from build123d import *

# Parameters (mm, degrees)
EXTRUDE_1_DEPTH     = 1500
CUT_EXTRUDE_4_DEPTH = 1500
SHELL_3_T           = 10


with BuildPart() as part:
    # 草图2 → 凸台-拉伸1 (new body)
    with BuildSketch(Plane(origin=(0, 0, 0), x_dir=(1, 0, 0), z_dir=(0, 1, 0))):
        Polygon((345, 8.660254038), (180, 294.448637287), (165, 303.108891325), (-165, 303.108891325), (-180, 294.448637287), (-345, 8.660254038), (-345, -8.660254038), (-180, -294.448637287), (-165, -303.108891325), (165, -303.108891325), (180, -294.448637287), (345, -8.660254038), align=None)
    extrude(amount=EXTRUDE_1_DEPTH)

    # 草图5 → 切除-拉伸4 (cut)
    with BuildSketch(Plane(origin=(0, 0, 0), x_dir=(1, 0, 0), z_dir=(0, 1, 0))):
        with BuildLine():
            Line((165, 303.108891325), (16.245071573, 258.879313504))
            ThreePointArc((16.245071573, 258.879313504), (0, 256.515365505), (-16.245071573, 258.879313504))
            Line((-16.245071573, 258.879313504), (-165, 303.108891325))
            Line((-165, 303.108891325), (-165, 323.92213511))
            Line((-165, 323.92213511), (-16.245047342, 368.151648331))
            ThreePointArc((-16.245047342, 368.151648331), (0, 370.515589126), (16.245047342, 368.151648331))
            Line((16.245047342, 368.151648331), (165, 323.92213511))
            Line((165, 323.92213511), (165, 303.108891325))
        make_face()
        with BuildLine():
            Line((198.024797853, 304.855259179), (310.706156229, 198.14444785))
            ThreePointArc((310.706156229, 198.14444785), (320.875912682, 185.257794563), (326.951203571, 170.007200482))
            Line((326.951203571, 170.007200482), (363.024797853, 19.06687593))
            Line((363.024797853, 19.06687593), (345, 8.660254038))
            Line((345, 8.660254038), (232.318597795, 115.371012084))
            ThreePointArc((232.318597795, 115.371012084), (222.148822988, 128.257682752), (216.073526222, 143.50830142))
            Line((216.073526222, 143.50830142), (180, 294.448637287))
            Line((180, 294.448637287), (198.024797853, 304.855259179))
        make_face()
        with BuildLine():
            Line((363.024797853, -19.06687593), (326.951203571, -170.007200482))
            ThreePointArc((326.951203571, -170.007200482), (320.875912682, -185.257794563), (310.706156229, -198.14444785))
            Line((310.706156229, -198.14444785), (198.024797853, -304.855259179))
            Line((198.024797853, -304.855259179), (180, -294.448637287))
            Line((180, -294.448637287), (216.073526222, -143.50830142))
            ThreePointArc((216.073526222, -143.50830142), (222.148822988, -128.257682752), (232.318597795, -115.371012084))
            Line((232.318597795, -115.371012084), (345, -8.660254038))
            Line((345, -8.660254038), (363.024797853, -19.06687593))
        make_face()
        with BuildLine():
            Line((165, -323.92213511), (16.245047342, -368.151648331))
            ThreePointArc((16.245047342, -368.151648331), (0, -370.515589126), (-16.245047342, -368.151648331))
            Line((-16.245047342, -368.151648331), (-165, -323.92213511))
            Line((-165, -323.92213511), (-165, -303.108891325))
            Line((-165, -303.108891325), (-16.245071573, -258.879313504))
            ThreePointArc((-16.245071573, -258.879313504), (0, -256.515365505), (16.245071573, -258.879313504))
            Line((16.245071573, -258.879313504), (165, -303.108891325))
            Line((165, -303.108891325), (165, -323.92213511))
        make_face()
        with BuildLine():
            Line((-198.024797853, -304.855259179), (-310.706156229, -198.14444785))
            ThreePointArc((-310.706156229, -198.14444785), (-320.875912682, -185.257794563), (-326.951203571, -170.007200482))
            Line((-326.951203571, -170.007200482), (-363.024797853, -19.06687593))
            Line((-363.024797853, -19.06687593), (-345, -8.660254038))
            Line((-345, -8.660254038), (-232.318597795, -115.371012084))
            ThreePointArc((-232.318597795, -115.371012084), (-222.148822988, -128.257682752), (-216.073526222, -143.50830142))
            Line((-216.073526222, -143.50830142), (-180, -294.448637287))
            Line((-180, -294.448637287), (-198.024797853, -304.855259179))
        make_face()
        with BuildLine():
            Line((-363.024797853, 19.06687593), (-326.951203571, 170.007200482))
            ThreePointArc((-326.951203571, 170.007200482), (-320.875912682, 185.257794563), (-310.706156229, 198.14444785))
            Line((-310.706156229, 198.14444785), (-198.024797853, 304.855259179))
            Line((-198.024797853, 304.855259179), (-180, 294.448637287))
            Line((-180, 294.448637287), (-216.073526222, 143.50830142))
            ThreePointArc((-216.073526222, 143.50830142), (-222.148822988, 128.257682752), (-232.318597795, 115.371012084))
            Line((-232.318597795, 115.371012084), (-345, 8.660254038))
            Line((-345, 8.660254038), (-363.024797853, 19.06687593))
        make_face()
    extrude(amount=CUT_EXTRUDE_4_DEPTH, mode=Mode.SUBTRACT)

    # 抽壳3 (no face opened: a closed hollow body)
    add(offset(amount=-SHELL_3_T, mode=Mode.PRIVATE), mode=Mode.SUBTRACT)


solid = part.part
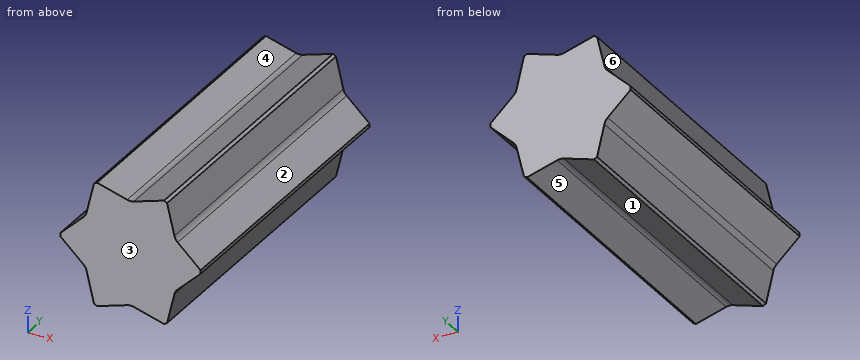
Geometry check sheet. Reference: the model listing, model coordinates, mm. Face numbers are marked on the shaded views. A direction names the side the tool comes from. Give positions to 0.01 mm unless a question says otherwise; leave off trailing zeros. Loops run counter-clockwise (first coordinate to the right, second up) from the corner with the lowest first, then second, coordinate; pieces in that order, holes last. Notation, with made-up numbers: (-20.75, 51) -> (10.25, 51) arc R19 cw to (10.25, 81) -> close; hole circle Ø9 at (-35.5, 28.5). An arc over 180 degrees is marked (long way). Answer in a Markdown table with one row per item. Add a question column.
1) Set-up check for the marked faces 4, 5 and 6: record each of +Z, -Z, +X, -X, +Y, -Y from which the full face is reachable in a straight line by a thin tool's end or side.
2) Cross-section at A-A on z = -216. Record the boundary of the cut face in (x, y).
3) Draft check along X on the marked faces 1, 2 and 3. Enter one of: pulls with the +X half, pulls with the -X half, needs draft (parallel to the pull), parting line crosses it, or undercut.
4) Cross-section at B-B on x = 144.5. Record the boundary of the cut face in (y, z), and give its area (3 significant figures).
5) Material ranges on probe 1 along Y at (x, z) = (-228.5, -64); probe 2 along X at (y, z) = (628, 4.5); probe 3 along X at (y, z) = (521, 136.5), recorded low to high. Write a range as from..to.
6) Gauge pin test, flat ends, axial feed: P1, Ø6, axis at y = 332.5, z = 13, coming from the +X side; P2, Ø1.5, axis at y = 405.5, z = -63, coming from the +X side; P3, Ø2, axis at x = 275.5, y = 230.5, coming from the +Z side. Record the tip position at first contact, or that the pin passes through.
Outcome:
| question | item | result |
|---|---|---|
| 1 | face 4 | +Z, +Y, -Y |
| 1 | face 5 | -Z, +Y, -Y |
| 1 | face 6 | +Z, -X, +Y, -Y |
| 2 | outline | (-198.75, 0) -> (198.75, 0) -> (198.75, 1500) -> (-198.75, 1500) -> close; hole (-188.47, 10) -> (188.47, 10) -> (188.47, 1490) -> (-188.47, 1490) -> close |
| 3 | face 1 | undercut |
| 3 | face 2 | pulls with the +X half |
| 3 | face 3 | needs draft |
| 4 | outline | (0, -297.01) -> (1500, -297.01) -> (1500, 297.01) -> (0, 297.01) -> close; hole (10, -286.58) -> (1490, -286.58) -> (1490, 286.58) -> (10, 286.58) -> close |
| 4 | area | 42,800 mm^2 |
| 5 | probe 1 | y = 0..10, 1490..1500 |
| 5 | probe 2 | x = -345..-334.85, 334.85..345 |
| 5 | probe 3 | x = -218.23..-207.65, 207.65..218.23 |
| 6 | P1 | stops at x = 343.59 |
| 6 | P2 | stops at x = 288.41 |
| 6 | P3 | stops at z = 75.42 |
